from build123d import *

# Parameters (mm, degrees)
F0_R     = 3.121691
F1_DEPTH = 20.574


with BuildPart() as f1:
    # F0 (on Front) → F1 (new body)
    with BuildSketch(Plane.XZ):
        with BuildLine():
            Line((0, 28.73937), (0, 42.082649))
            ThreePointArc((0, 42.082649), (-50.585156, 3.592419), (0, -34.897812))
            ThreePointArc((0, -34.897812), (7.803079, -28.230312), (0, -21.562812))
            ThreePointArc((0, -21.562812), (-34.431843, 3.588279), (0, 28.73937))
        make_face()
        with Locations((-9.494251, 35.924211)):
            Circle(F0_R, mode=Mode.SUBTRACT)
    extrude(amount=F1_DEPTH)


solid = f1.part
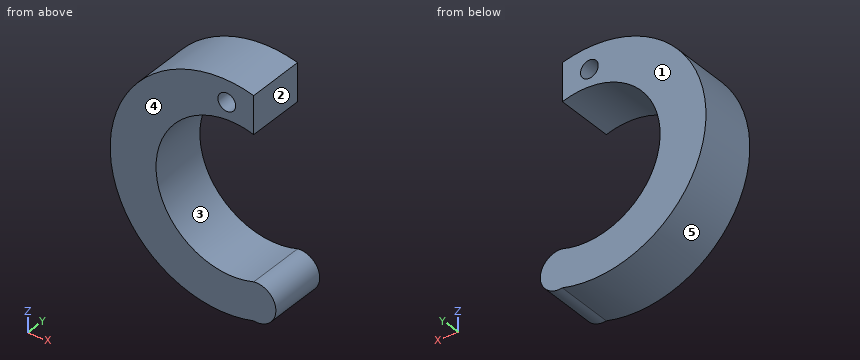
Model file for the job. Use its own axes, mm. Face numbers are marked on the shaded views. A direction names the side the tool comes from. Round coordinates to 2 decimals unless told otherwise and drop trailing zeros. Loops run counter-clockwise (first coordinate to the right, second up) from the corner with the lowest first, then second, coordinate; pieces in that order, holes last. Notation, with made-up numbers: (-11, 0.25) -> (-6, 0.25) arc R18 ccw to (-6, 14.25) -> close; hole circle Ø8 at (71.25, 1). An arc over 180 degrees is marked (long way). Answer as CSV lines item,"result". Start each with the question number.
1) Slice it at B-B (z = 37.5). List the corners of the cut face in (x, y), plus the area to 3 significant figures.
2) Slice it at C-C (y = -2.5). List the corners of the cut face in (x, z), plus the area to 3 significant figures.
3) Tool access for the marked faces 1 and 2: list every direction of +Z, -Z, +X, -X, +Y, -Y with a clear straight run to the whole face (end or side of a thin tool).
4) Probe line 1 along Z through (x, y) = (-22, -16.5); line 2 along X through (y, z) = (-4.5, 4.5); line 3 along Z through (x, y) = (-10, -5.25). List the from-to ranges inside material, lowest first.
5) Slice it at D-D (x = -38). List the corners of the cut face in (y, z), plus the area to 3 significant figures.
6) Pin check, flat tips, straight feed: P1, Ø10, axis at x = -33.5, y = -2.5, coming from the +Z side; P2, Ø2, axis at x = -15.5, y = -14, coming from the -Z side; P3, Ø6.5, axis at y = -7.5, z = 36.5, coming from the +X side. Stop position of each tip, or through.
7) Slice it at A-A (x = -3.5). List the corners of the cut face in (y, z).
8) Mould opens along Z. For the marked faces 3, 4 and 5 say: +Z half, -Z half, draft (parallel to the pull), parting line (faces both ways), or undercut.
Filled in:
1,outline,"(-31.75, -20.57) -> (-12.19, -20.57) -> (-12.19, 0) -> (-31.75, 0) -> close; (-6.8, -20.57) -> (0, -20.57) -> (0, 0) -> (-6.8, 0) -> close"
1,area,"542 mm2"
2,outline,"(0, -34.9) arc R6.75 ccw (long way) to (0, -21.56) arc R26.4 cw (long way) to (0, 28.74) -> (0, 42.08) arc R39.94 ccw (long way) to start; hole circle Ø6.24 at (-9.49, 35.92)"
2,area,"1,890 mm2"
3,face 1,"+Z, -Z, +X, -X, +Y"
3,face 2,"+Z, +X, +Y, -Y"
4,line 1,"z = -34.7 to -18.81, 25.99 to 41.88"
4,line 2,"x = -50.57 to -34.42"
4,line 3,"z = -36.34 to -22.74, 29.92 to 32.84, 39 to 43.52"
5,outline,"(-20.57, -25.51) -> (0, -25.51) -> (0, 32.69) -> (-20.57, 32.69) -> close"
5,area,"1,200 mm2"
6,P1,"stops at z = 39.32"
6,P2,"stops at z = -36.16"
6,P3,"stops at x = 0"
7,outline,"(-20.57, -35.7) -> (0, -35.7) -> (0, -22.42) -> (-20.57, -22.42) -> close; (-20.57, 29.6) -> (0, 29.6) -> (0, 42.88) -> (-20.57, 42.88) -> close"
8,face 3,"undercut"
8,face 4,"draft"
8,face 5,"parting line"
